Read the model definition and answer for the solid it produces. Units are mm, in the model's axes. Coordinates: 2 decimals unless noted, no trailing zeros. Order: outer loops, then holes, each group sorted by start corner. A loop starts at its lowest first (then second) coordinate and runs counter-clockwise, first axis right, second up. Notation, with made-up numbers: (31.5, 60) - (62.5, 60) arc R18 ccw to (62.5, 70) - close; hole circle Ø11 at (84, 43.5). An arc over 180 degrees is marked (long way). Use one line per item in the form item = value.
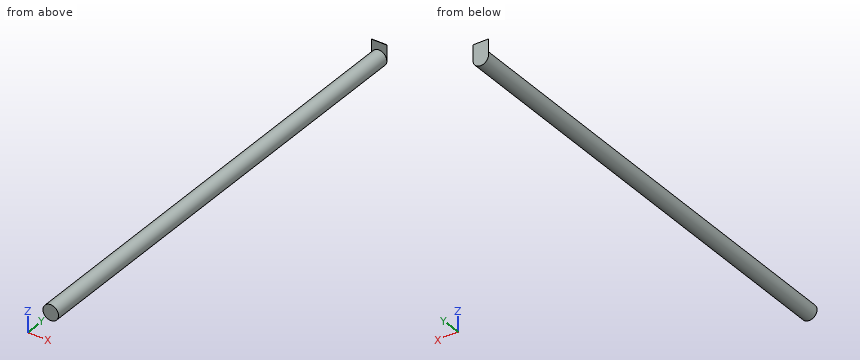
```python
from build123d import *

# Parameters (mm, degrees)
F0_R      = 6.35
F1_DEPTH  = 127
F1_FACE_R = 6.35
F2_DEPTH  = 254
F4_DEPTH  = 0.254


with BuildPart() as f1:
    # F0 (on Front) → F1 (new body)
    with BuildSketch(Plane.XZ):
        Circle(F0_R)
    extrude(amount=F1_DEPTH)

    # F1_face (on face) → F2 (join)
    with BuildSketch(Plane(origin=(0, 0, 0), x_dir=(1, 0, 0), z_dir=(0, 1, 0))):
        Circle(F1_FACE_R)
    extrude(amount=F2_DEPTH)

    # F3 (on face) → F4 (join)
    with BuildSketch(Plane(origin=(0, 254, 0), x_dir=(-1, 0, 0), z_dir=(0, 1, 0))):
        with BuildLine():
            Line((6.35, 12.7), (-6.35, 12.7))
            Line((-6.35, 12.7), (-6.35, 0))
            ThreePointArc((-6.35, 0), (0, 6.35), (6.35, 0))
            Line((6.35, 0), (6.35, 12.7))
        make_face()
    extrude(amount=-F4_DEPTH)


solid = f1.part
```
(1) Section B-B, the plane y = -53 is taken. Write down the section's boundary in (x, z).
Answer list:
outline = circle Ø12.7 at (0, 0)
(2) Straight lines are drawn through the part: L1, parallel to Y at x = 5.5, z = 4.25; L2, parallel to Z at x = -0.75, y = -88.5; L3, parallel to Z at x = -5, y = 170.5. For each, find the intervals that lie inside material, in ascending order.
Answer list:
L1 = 253.75 to 254
L2 = -6.31 to 6.31
L3 = -3.91 to 3.91
(3) Given pin 1 Ø1.5 at (y, z) = (51.5, 3.5) entering from +X; pin 2 Ø4 at (x, z) = (-2, 6.5) entering from -Y, each flat-ended and moving along its own axis, determine where each tip first touches the part or whether it passes through.
Answer list:
pin_1 = 5.72
pin_2 = -127
(4) Section A-A, the plane x = 0 is taken. Write down the section's boundary in (y, z), then the cut area to 3 significant figures.
Answer list:
outline = (-127, -6.35) - (254, -6.35) - (254, 12.7) - (253.75, 12.7) - (253.75, 6.35) - (-127, 6.35) - close
area = 4,840 mm2
